Source: three-view drawing plus pictorial views. Frame: mm from the lowest corner of the part. Coordinates: 2 decimals unless noted, no trailing zeros. Order: outer loops, then holes, each group sorted by start corner. A loop starts at its lowest first (then second) coordinate and runs counter-clockwise, first axis right, second up. Notation, with made-up numbers: (13, -14.5) - (65, -14.5) arc R14 cw to (65, 2.5) - close; hole circle Ø2 at (1.25, -5). An arc over 180 degrees is marked (long way). Use a Markdown table: item, result. Add a question column.
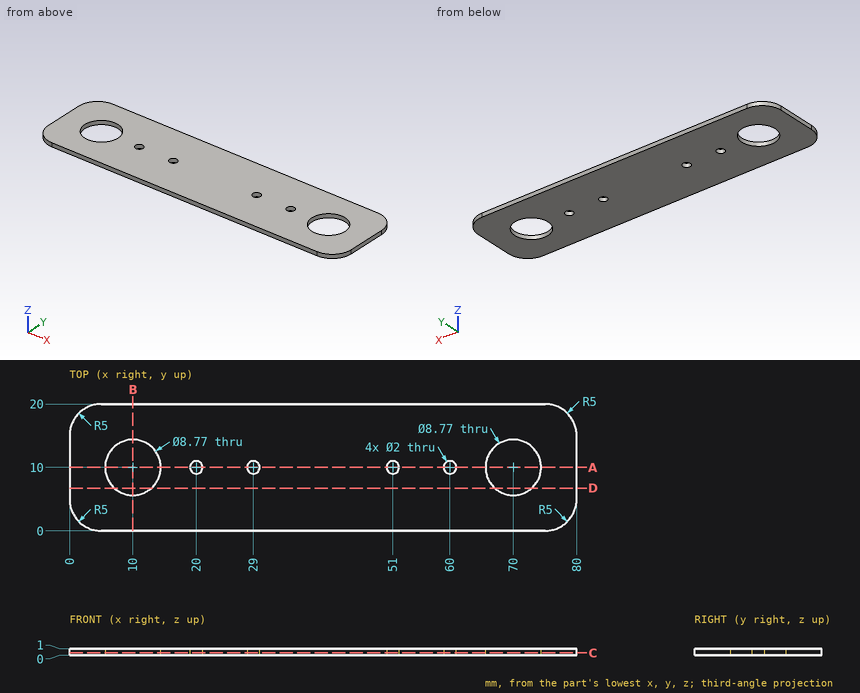
1) Section C-C (z = 0.35). Return loops of the section in (x, y) (3 decimals), then the cut area to 3 significant figures.
2) Section A-A (y = 10). Return loops of the section in (x, z) (3 decimals).
3) Section D-D (y = 6.75). Return loops of the section in (x, z), then the cut area to 3 significant figures.
4) Ray query, line 1 along X through (y, z) = (12.25, 0.6); line 2 along Y through (x, z) = (51, 0.85); line 3 along X through (y, z) = (8, 0.65). Return the intervals inside material, ascending.
5) Pin query (flat end, axial travel): pin 1 (8 mm diameter, centred on x = 70, y = 10, fed in from -Z). Return the tip coordinate at first contact, or that it passes through.
6) Section B-B (x = 10). Return loops of the section in (y, z) (3 decimals).
Values follow:
| question | item | result |
|---|---|---|
| 1 | outline | (0, 5) arc R5 ccw to (5, 0) - (75, 0) arc R5 ccw to (80, 5) - (80, 15) arc R5 ccw to (75, 20) - (5, 20) arc R5 ccw to (0, 15) - close; hole circle Ø8.77 at (10, 10); hole circle Ø2 at (20, 10); hole circle Ø2 at (29, 10); hole circle Ø2 at (51, 10); hole circle Ø2 at (60, 10); hole circle Ø8.77 at (70, 10) |
| 1 | area | 1,450 mm² |
| 2 | outline | (0, 0) - (5.615, 0) - (5.615, 1) - (0, 1) - close; (14.385, 0) - (19, 0) - (19, 1) - (14.385, 1) - close; (21, 0) - (28, 0) - (28, 1) - (21, 1) - close; (30, 0) - (50, 0) - (50, 1) - (30, 1) - close; (52, 0) - (59, 0) - (59, 1) - (52, 1) - close; (61, 0) - (65.615, 0) - (65.615, 1) - (61, 1) - close; (74.385, 0) - (80, 0) - (80, 1) - (74.385, 1) - close |
| 3 | outline | (0, 0) - (7.06, 0) - (7.06, 1) - (0, 1) - close; (12.94, 0) - (67.06, 0) - (67.06, 1) - (12.94, 1) - close; (72.94, 0) - (80, 0) - (80, 1) - (72.94, 1) - close |
| 3 | area | 68.2 mm² |
| 4 | line 1 | x = 0 to 6.24, 13.76 to 66.24, 73.76 to 80 |
| 4 | line 2 | y = 0 to 9, 11 to 20 |
| 4 | line 3 | x = 0 to 6.1, 13.9 to 66.1, 73.9 to 80 |
| 5 | pin 1 | passes through |
| 6 | outline | (0, 0) - (5.615, 0) - (5.615, 1) - (0, 1) - close; (14.385, 0) - (20, 0) - (20, 1) - (14.385, 1) - close |
